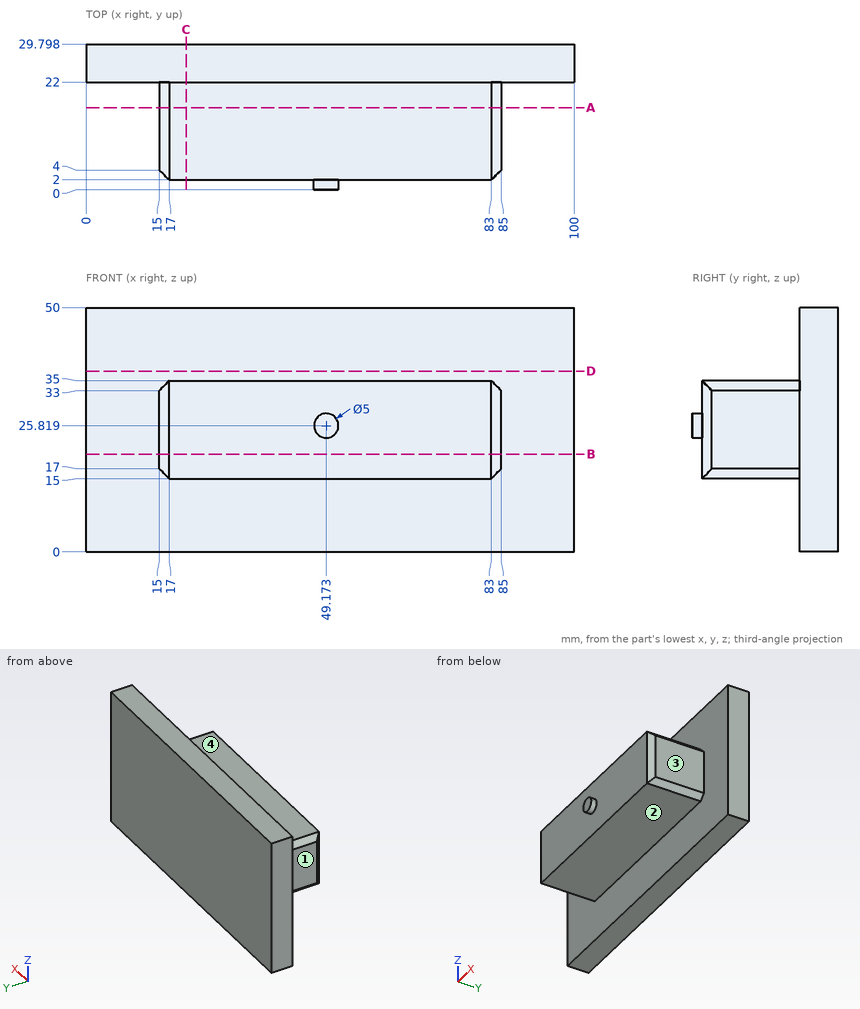
Input: dimensioned drawing with shaded views. Units: mm. Origin: part minimum x, y, z. A direction names the side the tool comes from. Coordinates: 2 decimals unless noted, no trailing zeros. Order: outer loops, then holes, each group sorted by start corner. A loop starts at its lowest first (then second) coordinate and runs counter-clockwise, first axis right, second up. Notation, with made-up numbers: (38.25, 10) -> (49.25, 10) arc R22 cw to (49.25, 45) -> close; hole circle Ø5 at (-5, 84.25). An arc over 180 degrees is marked (long way). Answer in a Markdown table with one row per item.
Item 1: Section D-D on z = 37. Output: boundary loops of the cut face in (x, y), plus the area to 3 significant figures.
Return value:
| item | result |
|---|---|
| outline | (0, 22) -> (100, 22) -> (100, 29.8) -> (0, 29.8) -> close |
| area | 780 mm² |
Item 2: Access query for the marked faces 1, 2, 3 and 4. Directions: +Z, -Z, +X, -X, +Y, -Y. A direction counts if a zero-diameter tool reaches every point of the face in a straight line with its end or side. Return the directions, or none.
Return value:
| item | result |
|---|---|
| face 1 | +Z, -Z, -X, -Y |
| face 2 | -Z, +X, -X, -Y |
| face 3 | +Z, -Z, +X, -Y |
| face 4 | +Z, +X, -X, -Y |
Item 3: Contact query for flat-ended pins moving along their axis: P1, Ø15, axis at x = 45.5, z = 19, coming from the -Y side; P2, Ø5, axis at y = 11, z = 23, coming from the -X side; P3, Ø13, axis at y = 14, z = 23.5, coming from the +X side; P4, Ø6, axis at x = 54.5, y = 9.5, coming from the +Z side. Output: stop coordinate, or through.
Return value:
| item | result |
|---|---|
| P1 | stops at y = 0 |
| P2 | stops at x = 15 |
| P3 | stops at x = 85 |
| P4 | stops at z = 35 |
Item 4: Section C-C on x = 20.5. Output: boundary loops of the cut face in (y, z).
Return value:
| item | result |
|---|---|
| outline | (2, 15) -> (22, 15) -> (22, 0) -> (29.8, 0) -> (29.8, 50) -> (22, 50) -> (22, 35) -> (2, 35) -> close |
Item 5: Ray query, L1, parallel to Y at x = 65, z = 47.5; L2, parallel to Z at x = 44.5, y = 15; L3, parallel to Y at x = 58, z = 23.5. Return the intervals inside material, ascending.
Return value:
| item | result |
|---|---|
| L1 | y = 22 to 29.8 |
| L2 | z = 15 to 35 |
| L3 | y = 2 to 29.8 |
Item 6: Section A-A on y = 16.75. Output: boundary loops of the cut face in (x, z).
Return value:
| item | result |
|---|---|
| outline | (15, 17) -> (17, 15) -> (83, 15) -> (85, 17) -> (85, 33) -> (83, 35) -> (17, 35) -> (15, 33) -> close |
Item 7: Section B-B on z = 20. Output: boundary loops of the cut face in (x, y), plus the area to 3 significant figures.
Return value:
| item | result |
|---|---|
| outline | (0, 22) -> (15, 22) -> (15, 4) -> (17, 2) -> (83, 2) -> (85, 4) -> (85, 22) -> (100, 22) -> (100, 29.8) -> (0, 29.8) -> close |
| area | 2,180 mm² |
